Could you check a few things on this drawing? It's one solid part, dimensions in mm from its lowest x, y, z. A direction names the side the tool comes from. Coordinates: 2 decimals unless noted, no trailing zeros. Loops run counter-clockwise (first coordinate to the right, second up) from the corner with the lowest first, then second, coordinate; pieces in that order, holes last. Notation, with made-up numbers: (47, 51.5) -> (95, 51.5) arc R18 ccw to (95, 65.5) -> close; hole circle Ø9 at (-28.75, 5.25). An arc over 180 degrees is marked (long way). One line per question, with ' | ' between items.
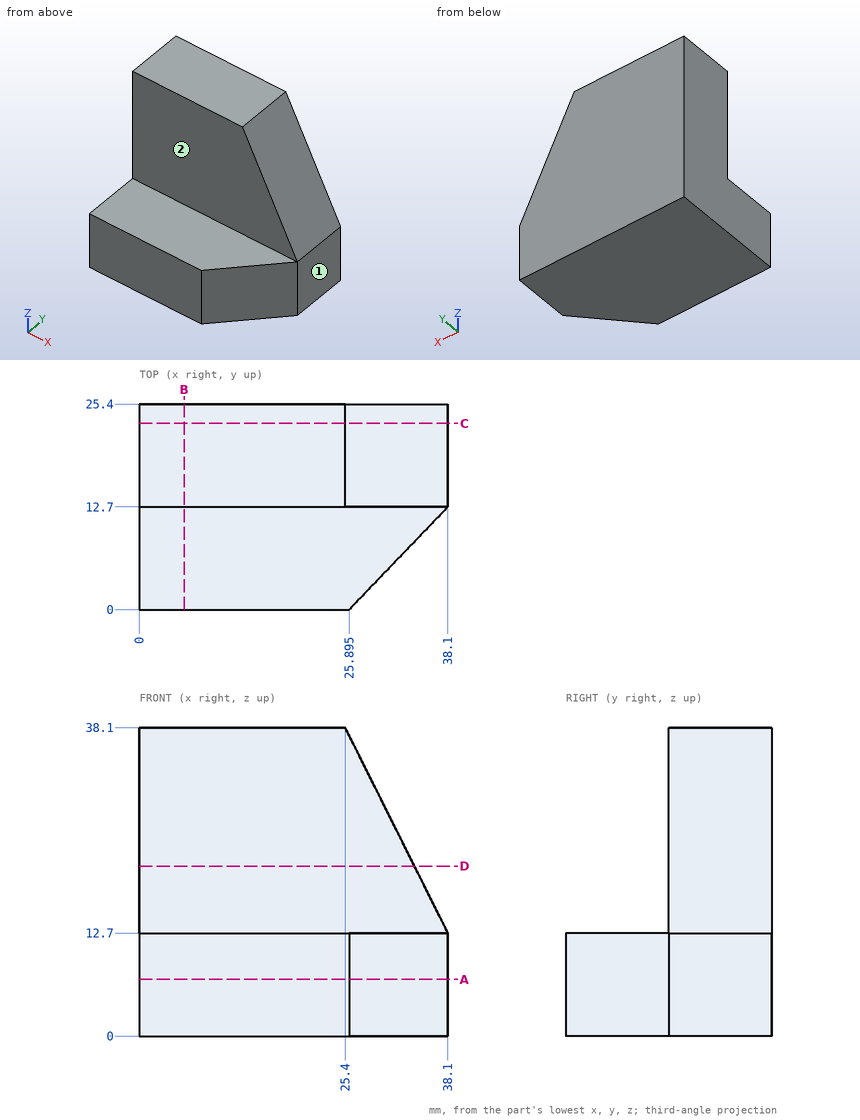
1) On a 3-axis mill with a long thin cutter (end or side, diameter ignored), from which of +Z, -Z, +X, -X, +Y, -Y can I reach the whole of each face in a straight line? I mean the marked faces 1 and 2. Say none if no direction works.
Data:
face 1: +Z, -Z, +X, +Y, -Y | face 2: +Z, +X, -X, -Y
2) I need wall thicknesses on line 1 along Y through (x, z) = (18.5, 27); line 2 along Z through (x, y) = (8, 5.75); line 3 along Z through (x, y) = (34.5, 14). Which ranges of each line are inside material? Lowest first, please. Write a range as from..to.
Data:
line 1: 12.7..25.4 | line 2: 0..12.7 | line 3: 0..19.9
3) If we section it at C-C on y = 23: Please give me the cut outline in (x, z), and give its area (3 significant figures).
Data:
outline: (0, 0) -> (38.1, 0) -> (38.1, 12.7) -> (25.4, 38.1) -> (0, 38.1) -> close | area: 1,290 mm²
4) I'm going to push flat-ended pins straight in: pin 1 Ø12 at (y, z) = (6, 24) entering from -X; pin 2 Ø12.5 at (x, z) = (25.5, 30) entering from -Y. Where does each tip first touch, or does it pass through?
Data:
pin 1: through | pin 2: y = 12.7
5) If we section it at A-A on z = 7: Please give me the cut outline in (x, y) (1 decimal), and give its area (3 significant figures).
Data:
outline: (0, 0) -> (25.9, 0) -> (38.1, 12.7) -> (38.1, 25.4) -> (0, 25.4) -> close | area: 890 mm²
6) If we section it at B-B on x = 5.5: Please give me the cut outline in (y, z), and give its area (3 significant figures).
Data:
outline: (0, 0) -> (25.4, 0) -> (25.4, 38.1) -> (12.7, 38.1) -> (12.7, 12.7) -> (0, 12.7) -> close | area: 645 mm²
7) If we section it at D-D on z = 21: Please give me the cut outline in (x, y), and give its area (3 significant figures).
Data:
outline: (0, 12.7) -> (33.95, 12.7) -> (33.95, 25.4) -> (0, 25.4) -> close | area: 431 mm²
